```python
from build123d import *

# Parameters (mm, degrees)
BOSS_EXTRUDE1_DEPTH = 10


with BuildPart() as part:
    # Sketch2 → Boss-Extrude1 (new body)
    with BuildSketch(Plane.XY):
        with BuildLine():
            Line((-200, 164.379500648), (-200, -15.620499352))
            Line((-200, -15.620499352), (-60, -15.620499352))
            ThreePointArc((-60, -15.620499352), (0, 62), (60, -15.620499352))
            Line((60, -15.620499352), (160, -15.620499352))
            Line((160, -15.620499352), (160, 164.379500648))
            Line((160, 164.379500648), (-200, 164.379500648))
        make_face()
    extrude(amount=BOSS_EXTRUDE1_DEPTH)


solid = part.part
```
For this review, take the finished solid that the model builds, in its own axes (mm). Round coordinates to 2 decimals unless told otherwise and drop trailing zeros. Loops run counter-clockwise (first coordinate to the right, second up) from the corner with the lowest first, then second, coordinate; pieces in that order, holes last.
(1) We need section C-C (x = 0). Give the boundary of the cut face in (y, z).
Returned:
outline: (62, 0) - (164.38, 0) - (164.38, 10) - (62, 10) - close
(2) Wall thickness on line 1 along X through (y, z) = (0, 7); line 2 along X through (y, z) = (51.5, 4.5); line 3 along Y through (x, z) = (55.5, 4.5): over which ranges is each line inside the solid? List them lowest first.
Returned:
line 1: x = -200 to -62, 62 to 160
line 2: x = -200 to -34.52, 34.52 to 160
line 3: y = 27.64 to 164.38
(3) We need section A-A (y = 0). Give the boundary of the cut face in (x, z).
Returned:
outline: (-200, 0) - (-62, 0) - (-62, 10) - (-200, 10) - close; (62, 0) - (160, 0) - (160, 10) - (62, 10) - close
(4) Mouldability with a two-part tool opening along X and no side actions: class faces 1 (the flat face through (-131, -15.62, 5)), 2 (the flat face through (-200, 76, 5)), 3 (the flat face through (160, 73, 5)), 4 (the cylindrical face through (-1.58, 61.98, 4.93)) as released by +X, released by -X, zero draft, split by the parting line, or undercut.
Returned:
face 1: zero draft
face 2: released by -X
face 3: released by +X
face 4: undercut
(5) We need section B-B (z = 2.75). Give the boundary of the cut face in (x, y).
Returned:
outline: (-200, -15.62) - (-60, -15.62) arc R62 cw (long way) to (60, -15.62) - (160, -15.62) - (160, 164.38) - (-200, 164.38) - close
(6) We need section D-D (x = 52). Give the boundary of the cut face in (y, z).
Returned:
outline: (33.76, 0) - (164.38, 0) - (164.38, 10) - (33.76, 10) - close
